Check sheet for the modelled part. Datum: model origin and axes. Units: mm. Round coordinates to 2 decimals unless told otherwise and drop trailing zeros. Loops run counter-clockwise (first coordinate to the right, second up) from the corner with the lowest first, then second, coordinate; pieces in that order, holes last. Notation, with made-up numbers: (-12, 62.5) -> (3, 62.5) arc R6 ccw to (3, 70.5) -> close; hole circle Ø9 at (-14.75, -25). An arc over 180 degrees is marked (long way). One line per question, with ' | ' between items.
```python
from build123d import *

# Parameters (mm, degrees)
BOSS_EXTRUDE1_DEPTH                               = 6.35
SKETCH7_W                                         = 6.35
SKETCH7_H                                         = 1.5875
CUT_EXTRUDE1_DEPTH                                = 90.479251261
CSK_FOR_6_FLAT_HEAD_MACHINE_SCREW_100_D           = 3.7973
CSK_FOR_6_FLAT_HEAD_MACHINE_SCREW_100_CSINK_D     = 7.0866
CSK_FOR_6_FLAT_HEAD_MACHINE_SCREW_100_CSINK_ANGLE = 100


with BuildPart() as part:
    # Sketch1 → Boss-Extrude1 (new body)
    with BuildSketch(Plane.XY):
        Polygon((-39.059416118, -2.212395735), (-39.059416118, 2.212395735), (-82.55, 6.095483582), (-82.55, -6.095483582), align=None)
        Polygon((39.059416118, -4.7625), (-39.059416118, -4.7625), (-74.619416118, -7.9375), (74.619416118, -7.9375), align=None)
        Polygon((-39.059416118, -4.7625), (-39.059416118, -2.212395735), (-82.55, -6.095483582), (-82.55, -6.35), (-85.400583882, -6.35), (-88.9, -6.662447868), (-88.9, -7.9375), (-74.619416118, -7.9375), align=None)
        Polygon((0, -1.275052132), (-14.280583882, 0), (-39.059416118, -2.212395735), (-39.059416118, -4.7625), align=None)
        Polygon((0, 1.275052132), (-39.059416118, 4.7625), (-39.059416118, 2.212395735), (-14.280583882, 0), align=None)
        Polygon((74.619416118, 7.9375), (-74.619416118, 7.9375), (-39.059416118, 4.7625), (39.059416118, 4.7625), align=None)
        Polygon((-74.619416118, 7.9375), (-88.9, 7.9375), (-88.9, 6.662447868), (-85.400583882, 6.35), (-82.55, 6.35), (-82.55, 6.095483582), (-39.059416118, 2.212395735), (-39.059416118, 4.7625), align=None)
        Polygon((39.059416118, -2.212395735), (14.280583882, 0), (0, -1.275052132), (39.059416118, -4.7625), align=None)
        Polygon((39.059416118, 2.212395735), (39.059416118, 4.7625), (0, 1.275052132), (14.280583882, 0), align=None)
        Polygon((14.280583882, 0), (0, 1.275052132), (-14.280583882, 0), (0, -1.275052132), align=None)
        Polygon((82.55, -6.095483582), (39.059416118, -2.212395735), (39.059416118, -4.7625), (74.619416118, -7.9375), (88.9, -7.9375), (88.9, -6.662447868), (85.400583882, -6.35), (82.55, -6.35), align=None)
        Polygon((88.9, 7.9375), (74.619416118, 7.9375), (39.059416118, 4.7625), (39.059416118, 2.212395735), (82.55, 6.095483582), (82.55, 6.35), (85.400583882, 6.35), (88.9, 6.662447868), align=None)
        Polygon((88.9, 6.35), (88.9, 6.662447868), (85.400583882, 6.35), align=None)
        Polygon((88.9, -6.35), (85.400583882, -6.35), (88.9, -6.662447868), align=None)
        Polygon((82.55, 6.095483582), (39.059416118, 2.212395735), (39.059416118, -2.212395735), (82.55, -6.095483582), align=None)
        Polygon((-88.9, -6.662447868), (-85.400583882, -6.35), (-88.9, -6.35), align=None)
        Polygon((-85.400583882, 6.35), (-88.9, 6.662447868), (-88.9, 6.35), align=None)
    extrude(amount=BOSS_EXTRUDE1_DEPTH)

    # Sketch4 → Tap Drill for #6-32 Tap1 (revolve, cut)
    with BuildSketch(Plane(origin=(-82.55, 0, 3.175), x_dir=(0, 0, 1), z_dir=(0, 1, 0))):
        Polygon((0, 0), (0, 13.51269403), (1.35255, 12.7), (1.35255, 0), align=None)
    tap_drill_for_6_32_tap1 = revolve(axis=Axis((-88.9, 0, 3.175), (1, 0, 0)), mode=Mode.SUBTRACT)

    # Mirror1: Tap Drill for #6-32 Tap1 across plane
    add(tap_drill_for_6_32_tap1.mirror(Plane(origin=(0, 0, 0), x_dir=(0, 0, 1), z_dir=(1, 0, 0))), mode=Mode.SUBTRACT)

    # Sketch5 → Tap Drill for #6-32 Tap2 (revolve, cut)
    with BuildSketch(Plane(origin=(-73.289583418, 7.9375, 3.175), x_dir=(0, 0, 1), z_dir=(1, 0, 0))):
        Polygon((0, 0), (0, 7.16269403), (1.35255, 6.35), (1.35255, 0), align=None)
    tap_drill_for_6_32_tap2 = revolve(axis=Axis((-73.289583418, 14.2875, 3.175), (0, -1, 0)), mode=Mode.SUBTRACT)

    # Mirror2: Tap Drill for #6-32 Tap2 across plane
    add(tap_drill_for_6_32_tap2.mirror(Plane(origin=(0, 0, 0), x_dir=(0, 0, 1), z_dir=(1, 0, 0))), mode=Mode.SUBTRACT)

    # Mirror3: Tap Drill for #6-32 Tap2 across plane
    add(tap_drill_for_6_32_tap2.mirror(Plane(origin=(0, 0, 0), x_dir=(0, 0, 1), z_dir=(0, -1, 0))), mode=Mode.SUBTRACT)

    # Mirror3 copy 1 sketch → Mirror3 copy 1 (revolve, cut)
    with BuildSketch(Plane(origin=(73.289583418, -7.9375, 3.175), x_dir=(0, 0, 1), z_dir=(-1, 0, 0))):
        Polygon((0, 0), (0, 7.16269403), (1.35255, 6.35), (1.35255, 0), align=None)
    revolve(axis=Axis((73.289583418, -14.2875, 3.175), (0, 1, 0)), mode=Mode.SUBTRACT)

    # Sketch7 → Cut-Extrude1 (cut, through all)
    with BuildSketch(Plane.XY.offset(6.35)):
        with Locations((-61.595, 7.14375)):
            Rectangle(SKETCH7_W, SKETCH7_H)
        with Locations((-61.595, -7.14375)):
            Rectangle(SKETCH7_W, SKETCH7_H)
        with Locations((61.595, -7.14375)):
            Rectangle(SKETCH7_W, SKETCH7_H)
        with Locations((61.595, 7.14375)):
            Rectangle(SKETCH7_W, SKETCH7_H)
    extrude(amount=-CUT_EXTRUDE1_DEPTH, mode=Mode.SUBTRACT)

    # CSK for #6 Flat Head Machine Screw (100)1 (through all)
    with Locations(Plane.XY.offset(6.35)):
        with Locations((-61.595, 0), (61.595, 0)):
            CounterSinkHole(CSK_FOR_6_FLAT_HEAD_MACHINE_SCREW_100_D / 2, CSK_FOR_6_FLAT_HEAD_MACHINE_SCREW_100_CSINK_D / 2, counter_sink_angle=CSK_FOR_6_FLAT_HEAD_MACHINE_SCREW_100_CSINK_ANGLE)


solid = part.part
```
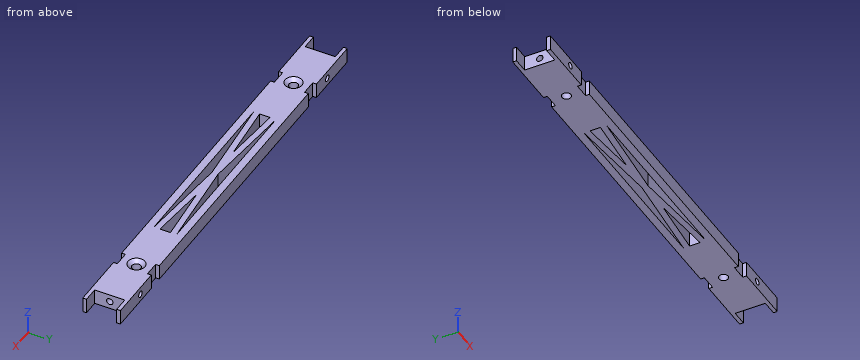
(1) Scan lines: probe 1 along X at (y, z) = (-7, 5); probe 2 along Z at (x, y) = (-74.5, 0); probe 3 along Y at (x, z) = (27.5, 5). Record each from-to range of solid material in increasing order.
Answer:
probe 1: x = -88.9 to -64.77, -58.42 to 58.42, 64.77 to 88.9 | probe 2: z = 0 to 1.82, 4.53 to 6.35 | probe 3: y = -7.94 to -4.76, -3.73 to -1.18, 1.18 to 3.73, 4.76 to 7.94
(2) Sectioned sample at B-B, the plane x = -28.5. Record the cut outline in (y, z).
Answer:
outline: (-7.94, 0) -> (-4.76, 0) -> (-4.76, 6.35) -> (-7.94, 6.35) -> close; (-3.82, 0) -> (-1.27, 0) -> (-1.27, 6.35) -> (-3.82, 6.35) -> close; (1.27, 0) -> (3.82, 0) -> (3.82, 6.35) -> (1.27, 6.35) -> close; (4.76, 0) -> (7.94, 0) -> (7.94, 6.35) -> (4.76, 6.35) -> close
(3) Go/stop test with flat-tipped pins: pin 1 (1.9 mm diameter, centred on y = -0.5, z = 4.5, fed in from +X); pin 2 (1 mm diameter, centred on y = -3.5, z = 5, fed in from -X); pin 3 (3 mm diameter, centred on x = 61, z = 4, fed in from +Y). Record where each tip stops, or that it passes through.
Answer:
pin 1: stops at x = 82.55 | pin 2: stops at x = -82.55 | pin 3: stops at y = 6.35
